Autodesk Inventor part; units mm, degrees
ref_plane "YZ Plane" through (0, 0, 0) normal (1, 0, 0) x (0, 1, 0)
ref_plane "XZ Plane" through (0, 0, 0) normal (0, 1, 0) x (-1, 0, 0)
ref_plane "XY Plane" through (0, 0, 0) normal (0, 0, 1) x (1, 0, 0)
sketch "スケッチ1" plane through (0, 0, 0) normal (1, 0, 0) x (0, 1, 0)
  line L0 (0, 0) -> (2.6147, 29.8858)
  line L1 (0, 0) -> (30, 0) construction
  line L2 (2.6147, 29.8858) -> (5.6147, 29.8858)
  line L3 (5.6147, 29.8858) -> (3, 0)
  line L4 (3, 0) -> (0, 0)
  dimension "d0" = 30
  dimension "d1" = 85
  dimension "d2" = 3
  dimension "d3" = 95
  dimension "d4" = 30
  dimension "d5" = 85
sketch "スケッチ2" plane through (0, 0, 0) normal (1, 0, 0) x (0, 1, 0)
  point P0 (0, 0)
extrude "押し出し1" add sketch "スケッチ1" along normal blind 150
sketch "スケッチ3" plane through (150, 0, 0) normal (1, 0, 0) x (0, 0, -1)
  line L0 (0, 0) -> (150, 0)
  line L1 (150, 0) -> (150, 3)
  line L2 (150, 3) -> (0, 3)
  line L3 (0, 3) -> (0, 0)
  dimension "d8" = 150
  dimension "d9" = 3
extrude "押し出し2" add sketch "スケッチ3" against normal blind 150
properties part number "NHK_t0_15"
Verification items for the finished model (mm, model axes). A direction names the side the tool comes from. Coordinates: 2 decimals unless noted, no trailing zeros. Write each loop counter-clockwise with the first axis right and the second up, starting at its lowest first coordinate (ties: lowest second). Pieces come first, ordered by that corner, then holes. Notation, with made-up numbers: (15, 16) - (69, 16) arc R4 ccw to (69, 20) - close; hole circle Ø4 at (59, 32). An arc over 180 degrees is marked (long way). Write item = value, one per line.
Q1. Cross-section at C-C (y = 4.45). Enter the section's corners in (x, z), plus the area to 3 significant figures.
Answer:
outline = (0, 16.57) - (150, 16.57) - (150, 29.89) - (0, 29.89) - close
area = 2,000 mm²
Q2. Cross-section at A-A (x = 50.5). Enter the section's corners in (y, z).
Answer:
outline = (0, -150) - (3, -150) - (3, 0) - (5.61, 29.89) - (2.61, 29.89) - (0, 0) - close
Q3. Cross-section at B-B (z = -104). Enter the section's corners in (x, y).
Answer:
outline = (0, 0) - (150, 0) - (150, 3) - (0, 3) - close
Q4. Go/stop test with a flat-tipped pin: pin 1 Ø10 at (x, z) = (26.5, -85.5) entering from +Y. Record where the tip stops, or that it passes through.
Answer:
pin_1 = 3
Q5. Access from +Z, -Z, +X, -X, +Y, -Y to the whole of each face (thin tool, end or side, straight path). Record for faces 1 (the face through (76, 3, -76)), 2 (the face through (0, 2, -59)).
Answer:
face_1 = -Z, +X, -X, +Y
face_2 = +Z, -Z, -X, +Y, -Y
Q6. Material ranges on L1, parallel to Y at x = 98, z = -104.5; L2, parallel to Y at x = 106, z = 16, recorded low to high. Write a range as from..to.
Answer:
L1 = 0..3
L2 = 1.4..4.4
